Verification items for the finished model (mm, model axes). A direction names the side the tool comes from. Give positions to 0.01 mm unless a question says otherwise; leave off trailing zeros.
from build123d import *

# Parameters (mm, degrees)
SKETCH1_W                    = 165
SKETCH1_H                    = 15
SKETCH2_R                    = 140
BOSS_EXTRUDE1_DEPTH          = 10
F_10_5_10_5_DIAMETER_HOLE1_D = 10.5
CHAMFER1_SIZE                = 1


with BuildPart() as part:
    # Sketch1 → Revolve1 (revolve)
    with BuildSketch(Plane.XZ, mode=Mode.PRIVATE) as revolve1_sk:
        with Locations((82.5, -7.5)):
            Rectangle(SKETCH1_W, SKETCH1_H)
    revolve(revolve1_sk.sketch.rotate(Axis((0, 0, 0), (0, 0, -1)), 180), axis=Axis((0, 0, 0), (0, 0, -1)))

    # Sketch2 → Boss-Extrude1 (add)
    with BuildSketch(Plane(origin=(0, 0, -15), x_dir=(-1, 0, 0), z_dir=(0, 0, -1))):
        Circle(SKETCH2_R)
    extrude(amount=BOSS_EXTRUDE1_DEPTH)

    # Sketch3 → Cut-Revolve1 (revolve, cut)
    with BuildSketch(Plane.XZ, mode=Mode.PRIVATE) as cut_revolve1_sk:
        Polygon((119, 0), (0, 0), (0, -25), (120, -25), (120, -10), (106, -10), (106, -2), (119, -2), align=None)
    revolve(cut_revolve1_sk.sketch.rotate(Axis((0, 0, 0), (0, 0, -1)), 180), axis=Axis((0, 0, 0), (0, 0, -1)), mode=Mode.SUBTRACT)

    # Sketch4 → Cut-Revolve2 (revolve, cut)
    with BuildSketch(Plane(origin=(0, -49.748846207, 0), x_dir=(1, 0, 0), z_dir=(0, 1, 0)), mode=Mode.PRIVATE) as cut_revolve2_sk:
        Polygon((-116.780839226, 25), (-120.104339226, 25), (-120.104339226, 10), (-116.780839226, 11.996960267), (-116.780839226, 15), align=None)
    revolve(cut_revolve2_sk.sketch.rotate(Axis((-120.104339226, -49.748846207, -25), (0, 0, 1)), 180), axis=Axis((-120.104339226, -49.748846207, -25), (0, 0, 1)), mode=Mode.SUBTRACT)

    # Sketch5 → Cut-Revolve3 (revolve, cut)
    with BuildSketch(Plane(origin=(0, -120.104339226, 0), x_dir=(1, 0, 0), z_dir=(0, 1, 0)), mode=Mode.PRIVATE) as cut_revolve3_sk:
        Polygon((-46.425346207, 25), (-49.748846207, 25), (-49.748846207, 10), (-46.425346207, 11.996960267), (-46.425346207, 15), align=None)
    revolve(cut_revolve3_sk.sketch.rotate(Axis((-49.748846207, -120.104339226, -25), (0, 0, 1)), 180), axis=Axis((-49.748846207, -120.104339226, -25), (0, 0, 1)), mode=Mode.SUBTRACT)

    # Sketch6 → Cut-Revolve4 (revolve, cut)
    with BuildSketch(Plane(origin=(0, -120.104339226, 0), x_dir=(1, 0, 0), z_dir=(0, 1, 0)), mode=Mode.PRIVATE) as cut_revolve4_sk:
        Polygon((53.072346207, 25), (49.748846207, 25), (49.748846207, 10), (53.072346207, 11.996960267), (53.072346207, 15), align=None)
    revolve(cut_revolve4_sk.sketch.rotate(Axis((49.748846207, -120.104339226, -25), (0, 0, 1)), 180), axis=Axis((49.748846207, -120.104339226, -25), (0, 0, 1)), mode=Mode.SUBTRACT)

    # Sketch7 → Cut-Revolve5 (revolve, cut)
    with BuildSketch(Plane(origin=(0, -49.748846207, 0), x_dir=(1, 0, 0), z_dir=(0, 1, 0)), mode=Mode.PRIVATE) as cut_revolve5_sk:
        Polygon((123.427839226, 25), (120.104339226, 25), (120.104339226, 10), (123.427839226, 11.996960267), (123.427839226, 15), align=None)
    revolve(cut_revolve5_sk.sketch.rotate(Axis((120.104339226, -49.748846207, -25), (0, 0, 1)), 180), axis=Axis((120.104339226, -49.748846207, -25), (0, 0, 1)), mode=Mode.SUBTRACT)

    # Sketch8 → Cut-Revolve6 (revolve, cut)
    with BuildSketch(Plane(origin=(0, 49.748846207, 0), x_dir=(1, 0, 0), z_dir=(0, 1, 0)), mode=Mode.PRIVATE) as cut_revolve6_sk:
        Polygon((123.427839226, 25), (120.104339226, 25), (120.104339226, 10), (123.427839226, 11.996960267), (123.427839226, 15), align=None)
    revolve(cut_revolve6_sk.sketch.rotate(Axis((120.104339226, 49.748846207, -25), (0, 0, 1)), 180), axis=Axis((120.104339226, 49.748846207, -25), (0, 0, 1)), mode=Mode.SUBTRACT)

    # Sketch9 → Cut-Revolve7 (revolve, cut)
    with BuildSketch(Plane(origin=(0, 120.104339226, 0), x_dir=(1, 0, 0), z_dir=(0, 1, 0)), mode=Mode.PRIVATE) as cut_revolve7_sk:
        Polygon((53.072346207, 25), (49.748846207, 25), (49.748846207, 10), (53.072346207, 11.996960267), (53.072346207, 15), align=None)
    revolve(cut_revolve7_sk.sketch.rotate(Axis((49.748846207, 120.104339226, -25), (0, 0, 1)), 180), axis=Axis((49.748846207, 120.104339226, -25), (0, 0, 1)), mode=Mode.SUBTRACT)

    # Sketch10 → Cut-Revolve8 (revolve, cut)
    with BuildSketch(Plane(origin=(0, 120.104339226, 0), x_dir=(1, 0, 0), z_dir=(0, 1, 0)), mode=Mode.PRIVATE) as cut_revolve8_sk:
        Polygon((-46.425346207, 25), (-49.748846207, 25), (-49.748846207, 10), (-46.425346207, 11.996960267), (-46.425346207, 15), align=None)
    revolve(cut_revolve8_sk.sketch.rotate(Axis((-49.748846207, 120.104339226, -25), (0, 0, 1)), 180), axis=Axis((-49.748846207, 120.104339226, -25), (0, 0, 1)), mode=Mode.SUBTRACT)

    # Sketch11 → Cut-Revolve9 (revolve, cut)
    with BuildSketch(Plane(origin=(0, 49.748846207, 0), x_dir=(1, 0, 0), z_dir=(0, 1, 0)), mode=Mode.PRIVATE) as cut_revolve9_sk:
        Polygon((-116.780839226, 25), (-120.104339226, 25), (-120.104339226, 10), (-116.780839226, 11.996960267), (-116.780839226, 15), align=None)
    revolve(cut_revolve9_sk.sketch.rotate(Axis((-120.104339226, 49.748846207, -25), (0, 0, 1)), 180), axis=Axis((-120.104339226, 49.748846207, -25), (0, 0, 1)), mode=Mode.SUBTRACT)

    # Ø10.5 (10.5) Diameter Hole1 (through all)
    with Locations(Plane(origin=(0, 0, -15), x_dir=(-1, 0, 0), z_dir=(0, 0, -1))):
        with Locations((152.5, 0), (107.833784131, -107.833784131), (0, -152.5), (-107.833784131, -107.833784131), (-152.5, 0), (-107.833784131, 107.833784131), (0, 152.5), (107.833784131, 107.833784131)):
            Hole(F_10_5_10_5_DIAMETER_HOLE1_D / 2)

    # Chamfer1
    chamfer1_edges = [part.edges().sort_by_distance(p)[0] for p in [
        (140, 0, -25),
        (120, 0, -25),
        (106, 0, -10),
        (106, 0, -2),
        (165, 0, -15),
        (165, 0, 0),
    ]]
    chamfer(chamfer1_edges, length=CHAMFER1_SIZE)


solid = part.part
(1) Go/stop test with flat-tipped pins: pin 1 (12 mm diameter, centred on x = 107.83, y = -107.83, fed in from -Z); pin 2 (1.5 mm diameter, centred on y = -28, z = -11, fed in from +X); pin 3 (3 mm diameter, centred on y = 110.5, z = -8.5, fed in from -X). Record where each tip stops, or that it passes through.
Solved:
pin 1: stops at z = -15
pin 2: stops at x = 162.73
pin 3: stops at x = -123.87
(2) Set-up check for faces 1 (the flat face through (72, 122, -15)), 2 (the cylindrical face through (-1.138, -157.625, -7.395)), 3 (the cylindrical face through (-113.505, 35.744, -0.986)): record each of +Z, -Z, +X, -X, +Y, -Y from which the full face is reachable in a straight line by a thin tool's end or side.
Solved:
face 1: -Z
face 2: +Z, -Z
face 3: +Z
(3) Scan lines: line 1 (Y direction, x = 2.5, z = -6); line 2 (Z direction, x = -103, y = -116); line 3 (Y direction, x = -104, z = -12.5). Record each from-to range of solid material in increasing order.
Solved:
line 1: y = -164.98 to -157.12, -147.88 to -105.97, 105.97 to 147.88, 157.12 to 164.98
line 2: z = -15 to 0
line 3: y = -128.1 to -111.42, -104.25 to -59.87, 59.87 to 104.25, 111.42 to 128.1
(4) Section check A-A, the plane y = 0. Give the number of separate pieces and of enclosed holes in the cut face, then the cut area to 3 significant figures.
Solved:
separate pieces: 4
enclosed holes: 0
area: 1,660 mm2
(5) Release check for a two-part mould opening along Y. For faces 4 (the cylindrical face through (-111.703, 111.382, -7.395)), 5 (the cylindrical face through (111.1, -85.19, -19.44)), 6 (the flat face through (-49, -109, 0)) record: pulls with the +Y half, pulls with the -Y half, needs draft (parallel to the pull), parting line crosses it, or undercut.
Solved:
face 4: undercut
face 5: parting line crosses it
face 6: needs draft
